For this review, take the finished solid that the model builds, in its own axes (mm). A direction names the side the tool comes from. Give positions to 0.01 mm unless a question says otherwise; leave off trailing zeros. Loops run counter-clockwise (first coordinate to the right, second up) from the corner with the lowest first, then second, coordinate; pieces in that order, holes last. Notation, with made-up numbers: (47, 77) - (59, 77) arc R20 cw to (59, 92) - close; hole circle Ø11 at (-31.5, 37). An arc over 180 degrees is marked (long way). Answer in a Markdown table with one row per item.
```python
from build123d import *

# Parameters (mm, degrees)
F0_R     = 16.51
F0_R_2   = 1.6129
F1_DEPTH = 12.7
F3_R     = 12.7
F3_R_2   = 1.6129
F2_R     = 12.7
F2_R_2   = 1.6129
F4_DEPTH = 1.27
F5_DEPTH = 1.27


# Not quite as in the source:
# - the program builds the solid bodies; features that only make, move or delete a surface that nothing else refers to are left out


with BuildPart() as f1:
    # F0 (on Front) → F1 (new body)
    with BuildSketch(Plane.XZ):
        with BuildLine():
            ThreePointArc((1.2694815268, 22.1887142857), (0, 23.495), (-1.2694815268, 22.1887142857))
            ThreePointArc((-1.2694815268, 22.1887142857), (-3.658114769, 21.9218799681), (-6.0039662348, 21.3986685205))
            ThreePointArc((-6.0039662348, 21.3986685205), (-7.628814029, 22.2219760938), (-8.405361267, 20.5742685647))
            ThreePointArc((-8.405361267, 20.5742685647), (-10.5779308102, 19.5463041206), (-12.6267910938, 18.2897449866))
            ThreePointArc((-12.6267910938, 18.2897449866), (-13.6508775395, 17.5386478213), (-14.6303896913, 16.730281602))
            ThreePointArc((-14.6303896913, 16.730281602), (-16.3514639147, 15.0525829294), (-17.8813072129, 13.1988437887))
            ThreePointArc((-17.8813072129, 13.1988437887), (-18.6060249794, 12.1559228143), (-19.2699883786, 11.0733090306))
            ThreePointArc((-19.2699883786, 11.0733090306), (-20.3530621849, 8.9276808129), (-21.1981062384, 6.6776430652))
            ThreePointArc((-21.1981062384, 6.6776430652), (-21.5449209105, 5.4559149517), (-21.8213848205, 4.2163716058))
            ThreePointArc((-21.8213848205, 4.2163716058), (-22.1490903571, 1.8353259531), (-22.2177615305, -0.5671838988))
            ThreePointArc((-22.2177615305, -0.5671838988), (-22.1490903571, -1.8353259531), (-22.0080956233, -3.0974751064))
            ThreePointArc((-22.0080956233, -3.0974751064), (-21.5449209105, -5.4559149517), (-20.8297776166, -7.7505476866))
            ThreePointArc((-20.8297776166, -7.7505476866), (-20.3530621849, -8.9276808129), (-19.8098877746, -10.0756623284))
            ThreePointArc((-19.8098877746, -10.0756623284), (-18.6060249794, -12.1559228143), (-17.1845640907, -14.0940193703))
            ThreePointArc((-17.1845640907, -14.0940193703), (-16.3514639147, -15.0525829294), (-15.4649712035, -15.9619951972))
            ThreePointArc((-15.4649712035, -15.9619951972), (-13.6508775395, -17.5386478213), (-11.6771363996, -18.9101853641))
            ThreePointArc((-11.6771363996, -18.9101853641), (-10.5779308102, -19.5463041206), (-9.4441850386, -20.1185982105))
            ThreePointArc((-9.4441850386, -20.1185982105), (-7.2164457031, -21.0207881968), (-4.9043097902, -21.6771393519))
            ThreePointArc((-4.9043097902, -21.6771393519), (-3.658114769, -21.9218799681), (-2.3999748833, -22.0950389355))
            ThreePointArc((-2.3999748833, -22.0950389355), (0, -22.225), (2.3999748833, -22.0950389355))
            ThreePointArc((2.3999748833, -22.0950389355), (3.658114769, -21.9218799681), (4.9043097902, -21.6771393519))
            ThreePointArc((4.9043097902, -21.6771393519), (7.2164457031, -21.0207881968), (9.4441850386, -20.1185982105))
            ThreePointArc((9.4441850386, -20.1185982105), (10.5779308102, -19.5463041206), (11.6771363996, -18.9101853641))
            ThreePointArc((11.6771363996, -18.9101853641), (13.6508775395, -17.5386478213), (15.4649712035, -15.9619951972))
            ThreePointArc((15.4649712035, -15.9619951972), (16.3514639147, -15.0525829294), (17.1845640907, -14.0940193703))
            ThreePointArc((17.1845640907, -14.0940193703), (18.6060249794, -12.1559228143), (19.8098877746, -10.0756623284))
            ThreePointArc((19.8098877746, -10.0756623284), (20.3530621849, -8.9276808129), (20.8297776166, -7.7505476866))
            ThreePointArc((20.8297776166, -7.7505476866), (21.5449209105, -5.4559149517), (22.0080956233, -3.0974751064))
            ThreePointArc((22.0080956233, -3.0974751064), (22.1490903571, -1.8353259531), (22.2177615305, -0.5671838988))
            ThreePointArc((22.2177615305, -0.5671838988), (22.1490903571, 1.8353259531), (21.8213848205, 4.2163716058))
            ThreePointArc((21.8213848205, 4.2163716058), (21.5449209105, 5.4559149517), (21.1981062384, 6.6776430652))
            ThreePointArc((21.1981062384, 6.6776430652), (20.3530621849, 8.9276808129), (19.2699883786, 11.0733090306))
            ThreePointArc((19.2699883786, 11.0733090306), (18.6060249794, 12.1559228143), (17.8813072129, 13.1988437887))
            ThreePointArc((17.8813072129, 13.1988437887), (16.3514639147, 15.0525829294), (14.6303896913, 16.730281602))
            ThreePointArc((14.6303896913, 16.730281602), (13.6508775395, 17.5386478213), (12.6267910938, 18.2897449866))
            ThreePointArc((12.6267910938, 18.2897449866), (10.5779308102, 19.5463041206), (8.405361267, 20.5742685647))
            ThreePointArc((8.405361267, 20.5742685647), (7.628814029, 22.2219760938), (6.0039662348, 21.3986685205))
            ThreePointArc((6.0039662348, 21.3986685205), (3.658114769, 21.9218799681), (1.2694815268, 22.1887142857))
        make_face()
        Circle(F0_R, mode=Mode.SUBTRACT)
        Circle(F0_R)
        Circle(F0_R_2, mode=Mode.SUBTRACT)
        with BuildLine():
            ThreePointArc((-19.2699883786, 11.0733090306), (-18.6060249794, 12.1559228143), (-17.8813072129, 13.1988437887))
            ThreePointArc((-17.8813072129, 13.1988437887), (-19.6692264068, 12.8505469751), (-19.2699883786, 11.0733090306))
        make_face()
        with BuildLine():
            ThreePointArc((-14.6303896913, 16.730281602), (-13.6508775395, 17.5386478213), (-12.6267910938, 18.2897449866))
            ThreePointArc((-12.6267910938, 18.2897449866), (-14.4309276846, 18.5408562683), (-14.6303896913, 16.730281602))
        make_face()
        with BuildLine():
            ThreePointArc((14.6303896913, 16.730281602), (14.4309276846, 18.5408562683), (12.6267910938, 18.2897449866))
            ThreePointArc((12.6267910938, 18.2897449866), (13.6508775395, 17.5386478213), (14.6303896913, 16.730281602))
        make_face()
        with BuildLine():
            ThreePointArc((19.2699883786, 11.0733090306), (19.6692264068, 12.8505469751), (17.8813072129, 13.1988437887))
            ThreePointArc((17.8813072129, 13.1988437887), (18.6060249794, 12.1559228143), (19.2699883786, 11.0733090306))
        make_face()
        with BuildLine():
            ThreePointArc((21.8213848205, 4.2163716058), (22.7760592482, 5.7676815204), (21.1981062384, 6.6776430652))
            ThreePointArc((21.1981062384, 6.6776430652), (21.5449209105, 5.4559149517), (21.8213848205, 4.2163716058))
        make_face()
        with BuildLine():
            ThreePointArc((22.0080956233, -3.0974751064), (23.4147526632, -1.9402017219), (22.2177615305, -0.5671838988))
            ThreePointArc((22.2177615305, -0.5671838988), (22.1490903571, -1.8353259531), (22.0080956233, -3.0974751064))
        make_face()
        with BuildLine():
            ThreePointArc((-21.8213848205, 4.2163716058), (-21.5449209105, 5.4559149517), (-21.1981062384, 6.6776430652))
            ThreePointArc((-21.1981062384, 6.6776430652), (-22.7760592482, 5.7676815204), (-21.8213848205, 4.2163716058))
        make_face()
        with BuildLine():
            ThreePointArc((-22.0080956233, -3.0974751064), (-22.1490903571, -1.8353259531), (-22.2177615305, -0.5671838988))
            ThreePointArc((-22.2177615305, -0.5671838988), (-23.4147526632, -1.9402017219), (-22.0080956233, -3.0974751064))
        make_face()
        with BuildLine():
            ThreePointArc((-19.8098877746, -10.0756623284), (-20.3530621849, -8.9276808129), (-20.8297776166, -7.7505476866))
            ThreePointArc((-20.8297776166, -7.7505476866), (-21.5160943098, -9.4378340022), (-19.8098877746, -10.0756623284))
        make_face()
        with BuildLine():
            ThreePointArc((-15.4649712035, -15.9619951972), (-16.3514639147, -15.0525829294), (-17.1845640907, -14.0940193703))
            ThreePointArc((-17.1845640907, -14.0940193703), (-17.2858332813, -15.9127305253), (-15.4649712035, -15.9619951972))
        make_face()
        with BuildLine():
            ThreePointArc((-9.4441850386, -20.1185982105), (-10.5779308102, -19.5463041206), (-11.6771363996, -18.9101853641))
            ThreePointArc((-11.6771363996, -18.9101853641), (-11.1823839994, -20.6632357846), (-9.4441850386, -20.1185982105))
        make_face()
        with BuildLine():
            ThreePointArc((-2.3999748833, -22.0950389355), (-3.658114769, -21.9218799681), (-4.9043097902, -21.6771393519))
            ThreePointArc((-4.9043097902, -21.6771393519), (-3.8671498986, -23.1745588234), (-2.3999748833, -22.0950389355))
        make_face()
        with BuildLine():
            ThreePointArc((2.3999748833, -22.0950389355), (3.8671498986, -23.1745588234), (4.9043097902, -21.6771393519))
            ThreePointArc((4.9043097902, -21.6771393519), (3.658114769, -21.9218799681), (2.3999748833, -22.0950389355))
        make_face()
        with BuildLine():
            ThreePointArc((9.4441850386, -20.1185982105), (11.1823839994, -20.6632357846), (11.6771363996, -18.9101853641))
            ThreePointArc((11.6771363996, -18.9101853641), (10.5779308102, -19.5463041206), (9.4441850386, -20.1185982105))
        make_face()
        with BuildLine():
            ThreePointArc((15.4649712035, -15.9619951972), (17.2858332813, -15.9127305253), (17.1845640907, -14.0940193703))
            ThreePointArc((17.1845640907, -14.0940193703), (16.3514639147, -15.0525829294), (15.4649712035, -15.9619951972))
        make_face()
        with BuildLine():
            ThreePointArc((19.8098877746, -10.0756623284), (21.5160943098, -9.4378340022), (20.8297776166, -7.7505476866))
            ThreePointArc((20.8297776166, -7.7505476866), (20.3530621849, -8.9276808129), (19.8098877746, -10.0756623284))
        make_face()
    extrude(amount=F1_DEPTH)

    # F3 (on face) + F2 (on face) → F4 (cut)
    with BuildSketch(Plane(origin=(0, 0, 0), x_dir=(-1, 0, 0), z_dir=(0, 1, 0))):
        Circle(F3_R)
        Circle(F3_R_2, mode=Mode.SUBTRACT)
    with BuildSketch(Plane.XZ.offset(12.7)):
        Circle(F2_R)
        Circle(F2_R_2, mode=Mode.SUBTRACT)
    extrude(amount=-F4_DEPTH, dir=(0, 1, 0), mode=Mode.SUBTRACT)

    # F2 (on face) → F5 (cut)
    with BuildSketch(Plane.XZ.offset(12.7)):
        Circle(F2_R)
    extrude(amount=-F5_DEPTH, mode=Mode.SUBTRACT)


solid = f1.part
```
1. Wall thickness on line 1 (Z direction, x = 0, y = -12.15) (3 decimals); line 2 (Z direction, x = 0, y = -9) (3 decimals); line 3 (Y direction, x = -0.5, z = 9.5): over which ranges is each line inside the solid? List them lowest first. Write a range as [from, to].
Values:
| item | result |
|---|---|
| line 1 | z = [-22.225, -12.7], [12.7, 23.495] |
| line 2 | z = [-22.225, -1.613], [1.613, 23.495] |
| line 3 | y = [-11.43, -1.27] |
2. For faces 4 (the face through (-0.034, -6.261, -22.225)), 5 (the face through (-3.62, -6.26, 21.93)), 6 (the face through (-17.3, -6.3, -15.9)), 7 (the face through (-22.146, -6.261, 1.869)), 8 (the face through (21.537, -6.261, -5.489)), list the 3-axis set-ups (+Z, -Z, +X, -X, +Y, -Y) from which the entire face can be reached by the end or side of a thin tool; tool diameter is ignored.
Values:
| item | result |
|---|---|
| face 4 | -Z, +Y, -Y |
| face 5 | +Z, +Y, -Y |
| face 6 | +Y, -Y |
| face 7 | -X, +Y, -Y |
| face 8 | +X, +Y, -Y |
3. We need section C-C, the plane z = 10. Give the boundary of the cut face in (x, y).
Values:
| item | result |
|---|---|
| outline | (-19.85, -12.7) - (-7.83, -12.7) - (-7.83, -11.43) - (7.83, -11.43) - (7.83, -12.7) - (19.85, -12.7) - (19.85, 0) - (7.83, 0) - (7.83, -1.27) - (-7.83, -1.27) - (-7.83, 0) - (-19.85, 0) - close |
4. Clearance check with flat-ended pins moving along their axes: pin 1 (4 mm diameter, centred on x = 0, z = 0, fed in from -Y); pin 2 (1.5 mm diameter, centred on x = 6, y = -7.5, fed in from -Z); pin 3 (7.5 mm diameter, centred on x = 0.5, z = -1.5, fed in from +Y). State where each tip first meets the part, or that it passes through.
Values:
| item | result |
|---|---|
| pin 1 | stops at y = -11.43 |
| pin 2 | stops at z = -21.6 |
| pin 3 | stops at y = -1.27 |
5. Mouldability with a two-part tool opening along Z and no side actions: class faces 1 (the face through (3.691, -6.261, 21.916)), 2 (the face through (10, 0, -10)), 3 (the face through (-21.53, -6.26, -9.41)) as released by +Z, released by -Z, zero draft, split by the parting line, or undercut.
Values:
| item | result |
|---|---|
| face 1 | released by +Z |
| face 2 | zero draft |
| face 3 | undercut |
6. We need section B-B, the plane z = 0. Give the boundary of the cut face in (x, y) (3 decimals), and give its area (3 significant figures).
Values:
| item | result |
|---|---|
| outline | (-22.225, -12.7) - (-12.7, -12.7) - (-12.7, -11.43) - (-1.613, -11.43) - (-1.613, -1.27) - (-12.7, -1.27) - (-12.7, 0) - (-22.225, 0) - close; (1.613, -11.43) - (12.7, -11.43) - (12.7, -12.7) - (22.225, -12.7) - (22.225, 0) - (12.7, 0) - (12.7, -1.27) - (1.613, -1.27) - close |
| area | 467 mm^2 |
7. We need section D-D, the plane x = -14. Give the boundary of the cut face in (y, z), and give its area (3 significant figures).
Values:
| item | result |
|---|---|
| outline | (-12.7, -17.26) - (0, -17.26) - (0, 18.76) - (-12.7, 18.76) - close |
| area | 457 mm^2 |
8. We need section A-A, the plane x = 0. Give the boundary of the cut face in (y, z) (3 decimals).
Values:
| item | result |
|---|---|
| outline | (-12.7, -22.225) - (0, -22.225) - (0, -12.7) - (-1.27, -12.7) - (-1.27, -1.613) - (-11.43, -1.613) - (-11.43, -12.7) - (-12.7, -12.7) - close; (-12.7, 12.7) - (-11.43, 12.7) - (-11.43, 1.613) - (-1.27, 1.613) - (-1.27, 12.7) - (0, 12.7) - (0, 23.495) - (-12.7, 23.495) - close |
